Could you check a few things on this drawing? It's one solid part, dimensions in mm from its lowest x, y, z. A direction names the side the tool comes from. Give positions to 0.01 mm unless a question says otherwise; leave off trailing zeros. Loops run counter-clockwise (first coordinate to the right, second up) from the corner with the lowest first, then second, coordinate; pieces in that order, holes last. Notation, with made-up numbers: (-35, -29.5) - (-8, -29.5) arc R33 cw to (-8, 6.5) - close; hole circle Ø6 at (61, 48.5). An arc over 180 degrees is marked (long way). Return JSON: item names as keys, results as strings. Group by question number.
(1) If we section it at D-D (z = 56.5): Please give me the cut outline in (x, y).
(2) If we section it at B-B (y = 9): Please give me the cut outline in (x, z) (3 decimals), then the cut area to 3 significant figures.
(3) On a 3-axis mill with a long thin cutter (end or side, diameter ignored), from which of +Z, -Z, +X, -X, +Y, -Y can I reach the whole of each face in a straight line? I mean the marked faces 1, 2 and 3. Say none if no direction works.
(4) For P1, Ø9.5, axis at x = 60, y = 6.5, coming from the +Z side; P2, Ø12, axis at x = 30, y = 25, coming from the +Z side; P3, Ø12, axis at x = 108.5, z = 56, coming from the -Y side, each with a flat end and sliding along its axis, tell me the tip position at first contact or that it passes through.
(5) If we section it at A-A (z = 20.5): Please give me the cut outline in (x, y) (3 decimals), then the cut area to 3 significant figures.
(6) I need wall thicknesses on probe 1 along Z at (x, y) = (93, 6.5); probe 2 along Z at (x, y) = (108, 17.5); probe 3 along Y at (x, z) = (20.5, 39.5). Which ranges of each line are inside material? Lowest first, please. Write a range as [from, to].
(7) If we section it at C-C (x = 88): Please give me the cut outline in (y, z), then the cut area to 3 significant figures.
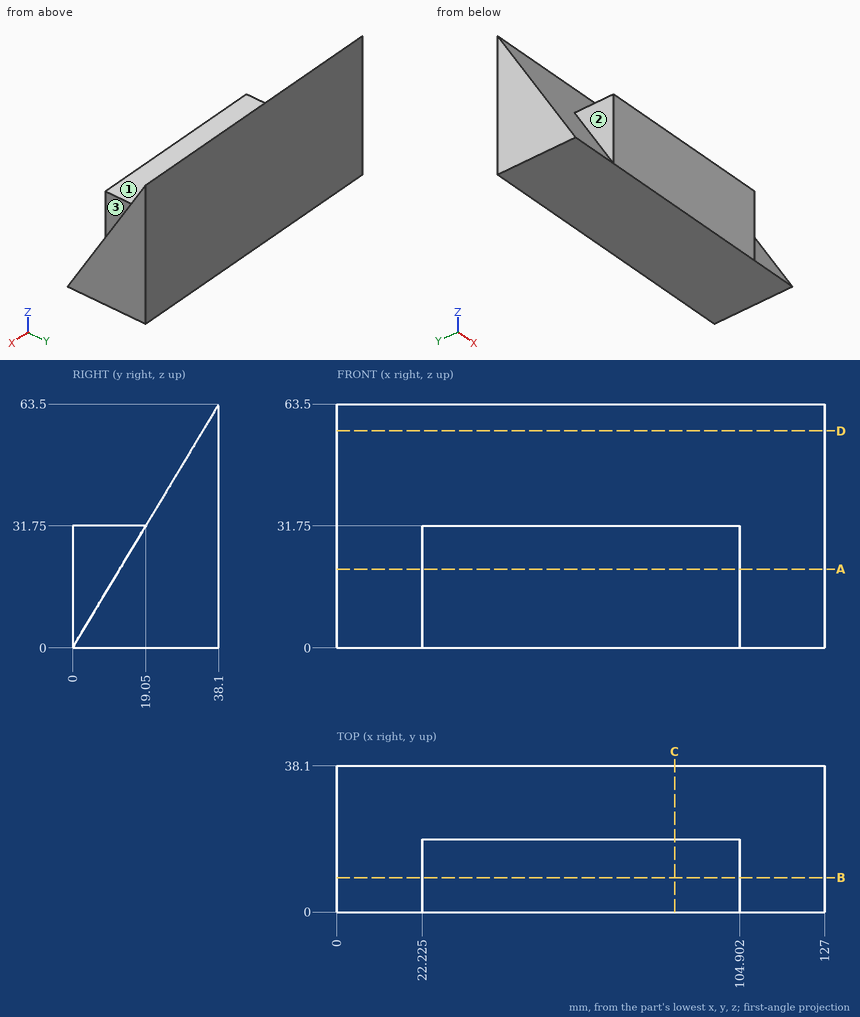
Values:
{
 "1": {"outline": "(0, 33.9) - (127, 33.9) - (127, 38.1) - (0, 38.1) - close"},
 "2": {"outline": "(0, 0) - (127, 0) - (127, 15) - (104.902, 15) - (104.902, 31.75) - (22.225, 31.75) - (22.225, 15) - (0, 15) - close", "area": "3,290 mm2"},
 "3": {"face 1": "+Z, +X, -X, -Y", "face 2": "+Z, -X, -Y", "face 3": "+Z, +X, -Y"},
 "4": {"P1": "z = 31.75", "P2": "z = 51.67", "P3": "y = 30"},
 "5": {"outline": "(0, 12.3) - (22.225, 12.3) - (22.225, 0) - (104.902, 0) - (104.902, 12.3) - (127, 12.3) - (127, 38.1) - (0, 38.1) - close", "area": "4,290 mm2"},
 "6": {"probe 1": "[0, 31.75]", "probe 2": "[0, 29.17]", "probe 3": "[23.7, 38.1]"},
 "7": {"outline": "(0, 0) - (38.1, 0) - (38.1, 63.5) - (19.05, 31.75) - (0, 31.75) - close", "area": "1,510 mm2"}
}
